Geometry: see drawing. Coordinates: mm, zero at the bounding-box minimum. A direction names the side the tool comes from. Coordinates: 2 decimals unless noted, no trailing zeros. Order: outer loops, then holes, each group sorted by start corner. A loop starts at its lowest first (then second) coordinate and runs counter-clockwise, first axis right, second up. Notation, with made-up numbers: (-18.75, 38.25) -> (-7.75, 38.25) arc R13 cw to (-7.75, 48.25) -> close; hole circle Ø1 at (-38, 52.5). An arc over 180 degrees is marked (long way). Use CSV: the item, a comma, the result in double quotes. Start each with the question number.
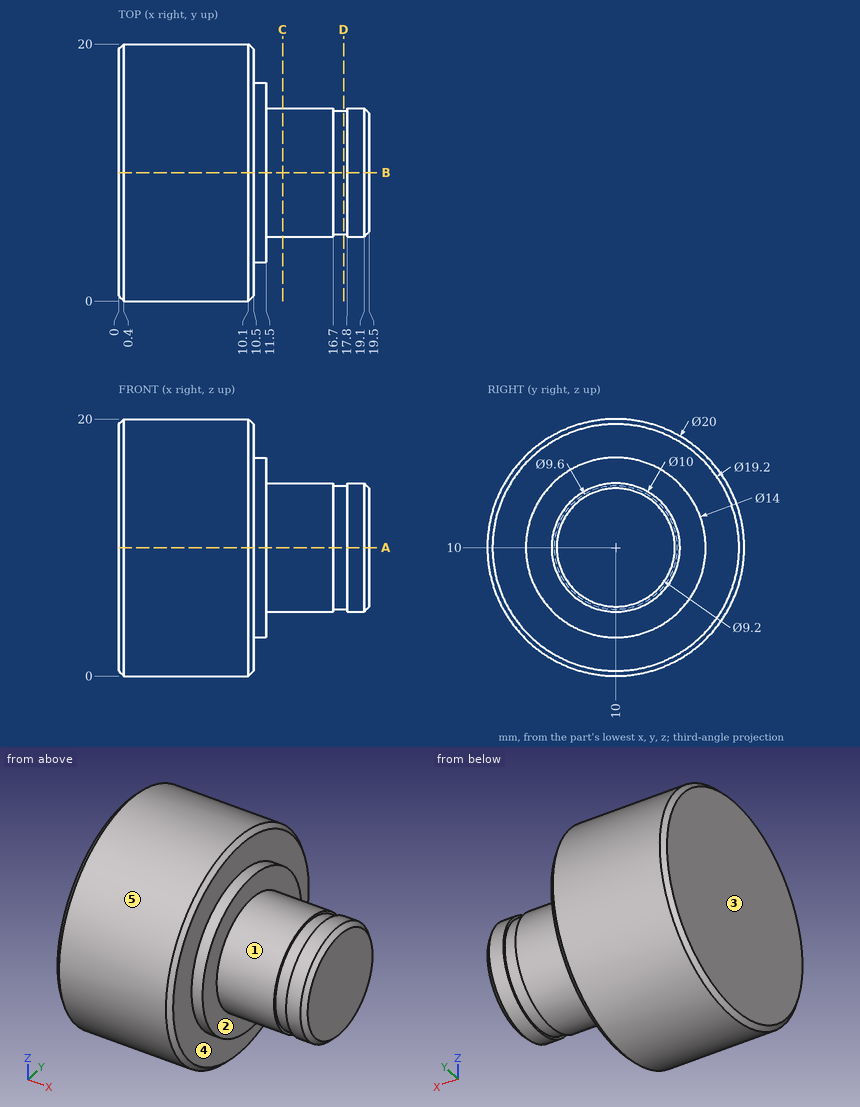
(1) Line query: line 1 (Y direction, x = 8.5, z = 10); line 2 (X direction, y = 7, z = 14.25); line 3 (X direction, y = 15.25, z = 17.5). Output: solid intervals per line, ascending. Write a range as from..to.
(2) Access query for the marked faces 4 and 5. Directions: +Z, -Z, +X, -X, +Y, -Y. A direction counts if a zero-diameter tool reaches every point of the face in a straight line with its end or side. Return the directions, or none.
(3) Section C-C (x = 12.75). Return loops of the section in (y, z), then the cut area to 3 significant figures.
(4) Section A-A (z = 10). Return loops of the section in (x, y), then the cut area to 3 significant figures.
(5) Section D-D (x = 17.5). Return loops of the section in (y, z), then the cut area to 3 significant figures.
(6) Mould query, pull axis X, two halves, no side actions, for the marked faces 1, 2 and 3. Classes: pulls with the +X half, pulls with the -X half, needs draft (parallel to the pull), parting line crosses it, or undercut.
(7) First-contact query: pin 1 (8 mm diameter, centred on x = 6, z = 15, fed in from +Y); pin 2 (1 mm diameter, centred on x = 5, y = 14.5, fed in from +Z); pin 3 (3 mm diameter, centred on y = 9, z = 11, fed in from -X); pin 4 (1.5 mm diameter, centred on x = 13, y = 15, fed in from -Z). Flat tips, straight axial feed; report the tip coordinate or a pass-through.
Check sheet entries:
1,line 1,"y = 0..20"
1,line 2,"x = 0..11.5"
1,line 3,"x = 0..10.5"
2,face 4,"+X"
2,face 5,"+X, -X"
3,outline,"circle Ø10 at (10, 10)"
3,area,"78.5 mm^2"
4,outline,"(0, 0.4) -> (0.4, 0) -> (10.1, 0) -> (10.5, 0.4) -> (10.5, 3) -> (11.5, 3) -> (11.5, 5) -> (16.7, 5) -> (16.7, 5.2) -> (17.8, 5.2) -> (17.8, 5) -> (19.1, 5) -> (19.5, 5.4) -> (19.5, 14.6) -> (19.1, 15) -> (17.8, 15) -> (17.8, 14.8) -> (16.7, 14.8) -> (16.7, 15) -> (11.5, 15) -> (11.5, 17) -> (10.5, 17) -> (10.5, 19.6) -> (10.1, 20) -> (0.4, 20) -> (0, 19.6) -> close"
4,area,"303 mm^2"
5,outline,"circle Ø9.6 at (10, 10)"
5,area,"72.4 mm^2"
6,face 1,"needs draft"
6,face 2,"pulls with the +X half"
6,face 3,"pulls with the -X half"
7,pin 1,"stops at y = 19.95"
7,pin 2,"stops at z = 19.17"
7,pin 3,"stops at x = 0"
7,pin 4,"stops at z = 7.37"
